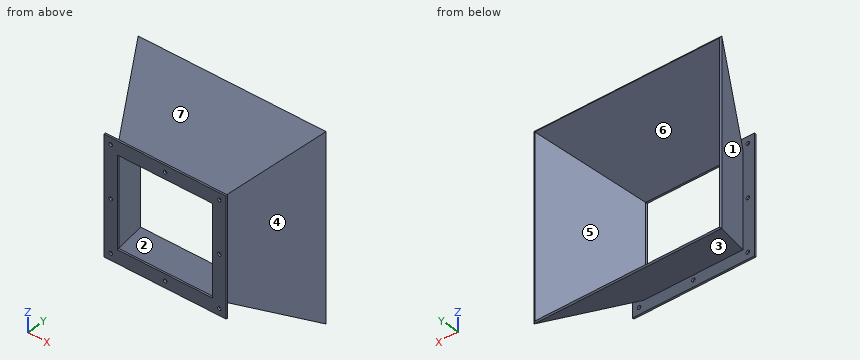
```python
from build123d import *

# Parameters (mm, degrees)
BOSS_EXTRUDE1_DEPTH   = 200
BOSS_EXTRUDE2_START   = -155
BOSS_EXTRUDE2_DEPTH   = 310
BOSS_EXTRUDE2_START_2 = 75
BOSS_EXTRUDE2_2_DEPTH = 77.598076211
CUT_EXTRUDE1_DEPTH    = 286.853377845
SKETCH4_W             = 315.196152422
SKETCH4_H             = 3
CUT_EXTRUDE2_DEPTH    = 373.124552005
SKETCH5_W             = 205
SKETCH5_H             = 22.5
BOSS_EXTRUDE3_DEPTH   = 3
SKETCH6_R             = 3
CUT_EXTRUDE3_DEPTH    = 255.947693633


with BuildPart() as part:
    # Sketch1 → Boss-Extrude1 (new, symmetric)
    with BuildSketch(Plane.XY):
        Polygon((-102.5, 0), (-102.5, -3), (-80, -3), (-80, 0), (-155, 129.903810568), (-157.598076211, 128.403810568), (-83.464101615, 0), align=None)
    extrude(amount=BOSS_EXTRUDE1_DEPTH, both=True)


with BuildPart() as body_2:
    # Mirror3: mirrored copy
    add(part.part.mirror(Plane(origin=(0, 0, 0), x_dir=(0, 0, 1), z_dir=(1, 0, 0))))


with BuildPart() as body_3:
    # Boss-Extrude2: read off the stored shape, not the designer's step
    # Boss-Extrude2 outline → Boss-Extrude2 (new body)
    with BuildSketch(Plane(origin=(0, 0, 0), x_dir=(0, 0, -1), z_dir=(1, 0, 0)).offset(BOSS_EXTRUDE2_START)):
        Polygon((-150, 129.903810568), (-152.598076211, 128.403810568), (-78.464101615, 0), (-97.5, 0), (-97.5, -3), (-75, -3), (-75, 0), align=None)
    extrude(amount=BOSS_EXTRUDE2_DEPTH)

    # Boss-Extrude2 2 outline → Boss-Extrude2 2 (cut)
    with BuildSketch(Plane.XY.offset(BOSS_EXTRUDE2_START_2)):
        Polygon((155, 129.903810568), (78.267949192, -3), (155, -3), align=None)
        Polygon((-155, 129.903810568), (-155, -3), (-78.267949192, -3), align=None)
    extrude(amount=BOSS_EXTRUDE2_2_DEPTH, mode=Mode.SUBTRACT)


with BuildPart() as body_4:
    # Mirror5: mirrored copy
    add(body_3.part.mirror(Plane.XY))


with BuildPart() as cut_extrude1_tool:
    # Sketch3 → Cut-Extrude1 (new, symmetric)
    with BuildSketch(Plane(origin=(0, 0, 0), x_dir=(0, 0, -1), z_dir=(1, 0, 0))):
        Polygon((-152.598076211, 128.403810568), (-78.464101615, 0), (-97.5, 0), (-97.5, -3), (-200, -3), (-200, 129.903810568), (-153.464101615, 129.903810568), align=None)
    cut_extrude1 = extrude(amount=CUT_EXTRUDE1_DEPTH, both=True)


with BuildPart() as part_1:
    add(part.part)

    # Cut-Extrude1: cut by cut_extrude1_tool
    add(cut_extrude1_tool.part, mode=Mode.SUBTRACT)


with BuildPart() as body_2_1:
    add(body_2.part)

    # Cut-Extrude1: cut by cut_extrude1_tool
    add(cut_extrude1_tool.part, mode=Mode.SUBTRACT)


with BuildPart() as cut_extrude2_tool:
    # Sketch4 → Cut-Extrude2 (new, through all)
    with BuildSketch(Plane(origin=(0, 162.37976321, 93.75), x_dir=(1, 0, 0), z_dir=(0, 0.8660254037844436, 0.4999999999999916))):
        with Locations((0, -66.451905284)):
            Rectangle(SKETCH4_W, SKETCH4_H)
    cut_extrude2 = extrude(amount=CUT_EXTRUDE2_DEPTH)


with BuildPart() as part_2:
    add(part_1.part)

    # Cut-Extrude2: cut by cut_extrude2_tool
    add(cut_extrude2_tool.part, mode=Mode.SUBTRACT)



with BuildPart() as body_2_2:
    add(body_2_1.part)

    # Cut-Extrude2: cut by cut_extrude2_tool
    add(cut_extrude2_tool.part, mode=Mode.SUBTRACT)


with BuildPart() as part_3:
    add(part_2.part)

    add(body_2_2.part)  # Boss-Extrude3 merges body 2

    add(body_3.part)  # Boss-Extrude3 merges body 3
    # Sketch5 → Boss-Extrude3 (add)
    with BuildSketch(Plane.XZ.offset(3)):
        with Locations((0, 86.25)):
            Rectangle(SKETCH5_W, SKETCH5_H)
    boss_extrude3 = extrude(amount=-BOSS_EXTRUDE3_DEPTH)

    # Mirror9: Cut-Extrude1, Cut-Extrude2 across plane
    add(cut_extrude1.mirror(Plane.XY), mode=Mode.SUBTRACT)
    add(cut_extrude2.mirror(Plane.XY), mode=Mode.SUBTRACT)

    # Mirror9 2: Boss-Extrude3 across plane
    add(boss_extrude3.mirror(Plane.XY))

    # Combine5: union body 4
    add(body_4.part)

    # Sketch6 → Cut-Extrude3 (cut, through all)
    with BuildSketch(Plane(origin=(0, 0, 0), x_dir=(1, 0, 0), z_dir=(0, 1, 0))):
        with Locations(Location((-91.25, 86.25, 0), (0, 0, 270))):
            Circle(SKETCH6_R)
        with Locations(Location((0, 86.25, 0), (0, 0, 270))):
            Circle(SKETCH6_R)
        with Locations(Location((91.25, 86.25, 0), (0, 0, 270))):
            Circle(SKETCH6_R)
        with Locations(Location((-91.25, 0, 0), (0, 0, 270))):
            Circle(SKETCH6_R)
        with Locations(Location((91.25, 0, 0), (0, 0, 270))):
            Circle(SKETCH6_R)
        with Locations(Location((91.25, -86.25, 0), (0, 0, 270))):
            Circle(SKETCH6_R)
        with Locations(Location((0, -86.25, 0), (0, 0, 270))):
            Circle(SKETCH6_R)
        with Locations(Location((-91.25, -86.25, 0), (0, 0, 270))):
            Circle(SKETCH6_R)
    extrude(amount=-CUT_EXTRUDE3_DEPTH, mode=Mode.SUBTRACT)


solid = part_3.part
```
Geometry check sheet. Reference: the model listing, model coordinates, mm. Face numbers are marked on the shaded views. A direction names the side the tool comes from. Coordinates: 2 decimals unless noted, no trailing zeros. Order: outer loops, then holes, each group sorted by start corner. A loop starts at its lowest first (then second) coordinate and runs counter-clockwise, first axis right, second up. Notation, with made-up numbers: (25.5, -14.5) - (36.5, -14.5) arc R24 cw to (36.5, 21.5) - close; hole circle Ø6 at (-40, 11). An arc over 180 degrees is marked (long way). Answer as a JSON object with one key per item and string values. Group by question number.
Item 1: Scan lines: probe 1 along X at (y, z) = (-1.85, 0); probe 2 along Z at (x, y) = (91, -1); probe 3 along X at (y, z) = (-1.9, -86.25). Record each from-to range of solid material in increasing order.
Item 2: Sectioned sample at A-A, the plane x = -26. Record the cut outline in (y, z).
Item 3: Tool access check on the marked faces 1, 2 and 3. Record the directions out of +Z, -Z, +X, -X, +Y, -Y that give a thin tool (end or side, any length) a straight path to the whole face; none if there is none.
Item 4: Sectioned sample at C-C, the plane y = 92. Record the cut outline in (x, z).
Item 5: Draft check along X on the marked faces 4, 5, 6 and 7. Enter one of: +X half, -X half, draft (parallel to the pull), parting line (faces both ways), or undercut.
Item 6: Depth check by flat-ended pin: pin 1 Ø3 at (x, z) = (94, -112.5) entering from +Y; pin 2 Ø10 at (x, z) = (-78, 52.5) entering from +Y; pin 3 Ø3.5 at (y, z) = (-1.5, 36.5) entering from -X. Enter the tip coordinate at first touch or a pass-through.
Item 7: Sectioned sample at B-B, the plane z = 53.5. Record the cut outline in (x, y).
Item 8: Sectioned sample at D-D, the plane x = -123. Record the cut outline in (y, z).
Resolved:
{
 "1": {"probe 1": "-102.5 to -94.25, -88.25 to -80, 80 to 88.25, 94.25 to 102.5", "probe 2": "-97.5 to -89.24, -83.26 to -2.99, 2.99 to 83.26, 89.24 to 97.5", "probe 3": "-102.5 to -94.25, -88.25 to -3, 3 to 88.25, 94.25 to 102.5"},
 "2": {"outline": "(-3, -97.5) - (0, -97.5) - (0, -78.46) - (128.4, -152.6) - (129.9, -150) - (0, -75) - (-3, -75) - close; (-3, 75) - (0, 75) - (129.9, 150) - (128.4, 152.6) - (0, 78.46) - (0, 97.5) - (-3, 97.5) - close"},
 "3": {"face 1": "+Z, -Z, -X", "face 2": "+Y", "face 3": "-Z, +X, -X"},
 "4": {"outline": "(-136.58, -131.58) - (136.58, -131.58) - (136.58, 131.58) - (-136.58, 131.58) - close; hole (-133.12, -128.12) - (133.12, -128.12) - (133.12, 128.12) - (-133.12, 128.12) - close"},
 "5": {"face 4": "+X half", "face 5": "undercut", "face 6": "undercut", "face 7": "draft"},
 "6": {"pin 1": "y = 67.55", "pin 2": "y = 5.2", "pin 3": "x = -102.5"},
 "7": {"outline": "(-157.6, 128.4) - (-83.46, 0) - (-102.5, 0) - (-102.5, -3) - (-80, -3) - (-80, 0) - (-155, 129.9) - close; (80, -3) - (102.5, -3) - (102.5, 0) - (83.46, 0) - (157.6, 128.4) - (155, 129.9) - (80, 0) - close"},
 "8": {"outline": "(68.48, -118) - (128.4, -152.6) - (129.9, -150) - (74.48, -118) - (74.48, 118) - (129.9, 150) - (128.4, 152.6) - (68.48, 118) - close"}
}
